For this review, take the finished solid that the model builds, in its own axes (mm). Face numbers are marked on the shaded views. A direction names the side the tool comes from. Coordinates: 2 decimals unless noted, no trailing zeros. Loops run counter-clockwise (first coordinate to the right, second up) from the corner with the lowest first, then second, coordinate; pieces in that order, holes last. Notation, with made-up numbers: M 43,26 L 98,26 A11 ccw 98,36 Z; hole C 28.5,61 d4. An arc over 180 degrees is marked long. Use one line per item in the form item = value.
```python
from build123d import *

# Parameters (mm, degrees)
F1_DEPTH = 12.7
F2_DEPTH = 25
F3_COUNT = 28
F5_R     = 0.381


with BuildPart() as f1:
    # F0 (on Top) → F1 (new body)
    with BuildSketch(Plane.XY):
        with BuildLine():
            ThreePointArc((0, 31.75), (-22.4506403027, -22.4506403027), (31.75, 0))
            ThreePointArc((31.75, 0), (24.9039389343, 19.6940682835), (7.3181054768, 30.895110167))
            Line((7.3181054768, 30.895110167), (0, 26.67))
            Line((0, 26.67), (0, 31.75))
        make_face()
        Polygon((0, 7.9189362922), (6.858, 3.9594681461), (6.858, -3.9594681461), (0, -7.9189362922), (-6.858, -3.9594681461), (-6.858, 3.9594681461), align=None, mode=Mode.SUBTRACT)
        with BuildLine():
            Line((0, 26.67), (7.3181054768, 30.895110167))
            ThreePointArc((7.3181054768, 30.895110167), (3.6839348663, 31.5355533311), (0, 31.75))
            Line((0, 31.75), (0, 26.67))
        make_face()
    extrude(amount=F1_DEPTH)


with BuildPart() as f2:
    # F0 (on Top) → F2 (new body)
    with BuildSketch(Plane.XY):
        with BuildLine():
            Line((0, 26.67), (7.3181054768, 30.895110167))
            ThreePointArc((7.3181054768, 30.895110167), (3.6839348663, 31.5355533311), (0, 31.75))
            Line((0, 31.75), (0, 26.67))
        make_face()
    extrude(amount=F2_DEPTH)


with BuildPart() as f3_1:
    # F3: instance of F2
    add(f2.part.rotate(Axis((0, 0, 0), (0, 0, -1)), 1 * 360 / F3_COUNT))


with BuildPart() as f3_2:
    # F3: instance of F2
    add(f2.part.rotate(Axis((0, 0, 0), (0, 0, -1)), 2 * 360 / F3_COUNT))


with BuildPart() as f3_3:
    # F3: instance of F2
    add(f2.part.rotate(Axis((0, 0, 0), (0, 0, -1)), 3 * 360 / F3_COUNT))


with BuildPart() as f3_4:
    # F3: instance of F2
    add(f2.part.rotate(Axis((0, 0, 0), (0, 0, -1)), 4 * 360 / F3_COUNT))


with BuildPart() as f3_5:
    # F3: instance of F2
    add(f2.part.rotate(Axis((0, 0, 0), (0, 0, -1)), 5 * 360 / F3_COUNT))


with BuildPart() as f3_6:
    # F3: instance of F2
    add(f2.part.rotate(Axis((0, 0, 0), (0, 0, -1)), 6 * 360 / F3_COUNT))


with BuildPart() as f3_7:
    # F3: instance of F2
    add(f2.part.rotate(Axis((0, 0, 0), (0, 0, -1)), 7 * 360 / F3_COUNT))


with BuildPart() as f3_8:
    # F3: instance of F2
    add(f2.part.rotate(Axis((0, 0, 0), (0, 0, -1)), 8 * 360 / F3_COUNT))


with BuildPart() as f3_9:
    # F3: instance of F2
    add(f2.part.rotate(Axis((0, 0, 0), (0, 0, -1)), 9 * 360 / F3_COUNT))


with BuildPart() as f3_10:
    # F3: instance of F2
    add(f2.part.rotate(Axis((0, 0, 0), (0, 0, -1)), 10 * 360 / F3_COUNT))


with BuildPart() as f3_11:
    # F3: instance of F2
    add(f2.part.rotate(Axis((0, 0, 0), (0, 0, -1)), 11 * 360 / F3_COUNT))


with BuildPart() as f3_12:
    # F3: instance of F2
    add(f2.part.rotate(Axis((0, 0, 0), (0, 0, -1)), 12 * 360 / F3_COUNT))


with BuildPart() as f3_13:
    # F3: instance of F2
    add(f2.part.rotate(Axis((0, 0, 0), (0, 0, -1)), 13 * 360 / F3_COUNT))


with BuildPart() as f3_14:
    # F3: instance of F2
    add(f2.part.rotate(Axis((0, 0, 0), (0, 0, -1)), 14 * 360 / F3_COUNT))


with BuildPart() as f3_15:
    # F3: instance of F2
    add(f2.part.rotate(Axis((0, 0, 0), (0, 0, -1)), 15 * 360 / F3_COUNT))


with BuildPart() as f3_16:
    # F3: instance of F2
    add(f2.part.rotate(Axis((0, 0, 0), (0, 0, -1)), 16 * 360 / F3_COUNT))


with BuildPart() as f3_17:
    # F3: instance of F2
    add(f2.part.rotate(Axis((0, 0, 0), (0, 0, -1)), 17 * 360 / F3_COUNT))


with BuildPart() as f3_18:
    # F3: instance of F2
    add(f2.part.rotate(Axis((0, 0, 0), (0, 0, -1)), 18 * 360 / F3_COUNT))


with BuildPart() as f3_19:
    # F3: instance of F2
    add(f2.part.rotate(Axis((0, 0, 0), (0, 0, -1)), 19 * 360 / F3_COUNT))


with BuildPart() as f3_20:
    # F3: instance of F2
    add(f2.part.rotate(Axis((0, 0, 0), (0, 0, -1)), 20 * 360 / F3_COUNT))


with BuildPart() as f3_21:
    # F3: instance of F2
    add(f2.part.rotate(Axis((0, 0, 0), (0, 0, -1)), 21 * 360 / F3_COUNT))


with BuildPart() as f3_22:
    # F3: instance of F2
    add(f2.part.rotate(Axis((0, 0, 0), (0, 0, -1)), 22 * 360 / F3_COUNT))


with BuildPart() as f3_23:
    # F3: instance of F2
    add(f2.part.rotate(Axis((0, 0, 0), (0, 0, -1)), 23 * 360 / F3_COUNT))


with BuildPart() as f3_24:
    # F3: instance of F2
    add(f2.part.rotate(Axis((0, 0, 0), (0, 0, -1)), 24 * 360 / F3_COUNT))


with BuildPart() as f3_25:
    # F3: instance of F2
    add(f2.part.rotate(Axis((0, 0, 0), (0, 0, -1)), 25 * 360 / F3_COUNT))


with BuildPart() as f3_26:
    # F3: instance of F2
    add(f2.part.rotate(Axis((0, 0, 0), (0, 0, -1)), 26 * 360 / F3_COUNT))


with BuildPart() as f3_27:
    # F3: instance of F2
    add(f2.part.rotate(Axis((0, 0, 0), (0, 0, -1)), 27 * 360 / F3_COUNT))


with BuildPart() as f1_1:
    add(f1.part)

    # F4: cut F2, F3_1, F3_2, F3_3, F3_4, F3_5, F3_6, F3_7, F3_8, F3_9, F3_10, F3_11, F3_12, F3_13, F3_14, F3_15, F3_16, F3_17, F3_18, F3_19, F3_20, F3_21, F3_23, F3_22, F3_24, F3_25, F3_26, F3_27
    add(f2.part, mode=Mode.SUBTRACT)
    add(f3_1.part, mode=Mode.SUBTRACT)
    add(f3_2.part, mode=Mode.SUBTRACT)
    add(f3_3.part, mode=Mode.SUBTRACT)
    add(f3_4.part, mode=Mode.SUBTRACT)
    add(f3_5.part, mode=Mode.SUBTRACT)
    add(f3_6.part, mode=Mode.SUBTRACT)
    add(f3_7.part, mode=Mode.SUBTRACT)
    add(f3_8.part, mode=Mode.SUBTRACT)
    add(f3_9.part, mode=Mode.SUBTRACT)
    add(f3_10.part, mode=Mode.SUBTRACT)
    add(f3_11.part, mode=Mode.SUBTRACT)
    add(f3_12.part, mode=Mode.SUBTRACT)
    add(f3_13.part, mode=Mode.SUBTRACT)
    add(f3_14.part, mode=Mode.SUBTRACT)
    add(f3_15.part, mode=Mode.SUBTRACT)
    add(f3_16.part, mode=Mode.SUBTRACT)
    add(f3_17.part, mode=Mode.SUBTRACT)
    add(f3_18.part, mode=Mode.SUBTRACT)
    add(f3_19.part, mode=Mode.SUBTRACT)
    add(f3_20.part, mode=Mode.SUBTRACT)
    add(f3_21.part, mode=Mode.SUBTRACT)
    add(f3_23.part, mode=Mode.SUBTRACT)
    add(f3_22.part, mode=Mode.SUBTRACT)
    add(f3_24.part, mode=Mode.SUBTRACT)
    add(f3_25.part, mode=Mode.SUBTRACT)
    add(f3_26.part, mode=Mode.SUBTRACT)
    add(f3_27.part, mode=Mode.SUBTRACT)

    # F5
    f5_edges = [f1_1.edges().sort_by_distance(p)[0] for p in [
        (-31.507862, 0, 6.35),
        (-30.717895, 7.011159, 6.35),
        (-28.387603, 13.670749, 6.35),
        (-24.633839, 19.644831, 6.35),
        (-19.644831, 24.633839, 6.35),
        (-13.670749, 28.387603, 6.35),
        (-7.011159, 30.717895, 6.35),
        (0, 31.507862, 6.35),
        (7.011159, 30.717895, 6.35),
        (13.670749, 28.387603, 6.35),
        (19.644831, 24.633839, 6.35),
        (24.633839, 19.644831, 6.35),
        (28.387603, 13.670749, 6.35),
        (30.717895, 7.011159, 6.35),
        (31.507862, 0, 6.35),
        (30.717895, -7.011159, 6.35),
        (28.387603, -13.670749, 6.35),
        (24.633839, -19.644831, 6.35),
        (19.644831, -24.633839, 6.35),
        (13.670749, -28.387603, 6.35),
        (7.011159, -30.717895, 6.35),
        (0, -31.507862, 6.35),
        (-7.011159, -30.717895, 6.35),
        (-13.670749, -28.387603, 6.35),
        (-19.644831, -24.633839, 6.35),
        (-24.633839, -19.644831, 6.35),
        (-28.387603, -13.670749, 6.35),
        (-30.717895, -7.011159, 6.35),
        (26.001327, 5.934633, 6.35),
        (26.67, 0, 6.35),
        (26.001327, -5.934633, 6.35),
        (24.02884, -11.571679, 6.35),
        (20.851446, -16.628473, 6.35),
        (16.628473, -20.851446, 6.35),
        (11.571679, -24.02884, 6.35),
        (5.934633, -26.001327, 6.35),
        (0, -26.67, 6.35),
        (-5.934633, -26.001327, 6.35),
        (-11.571679, -24.02884, 6.35),
        (-16.628473, -20.851446, 6.35),
        (-20.851446, -16.628473, 6.35),
        (-24.02884, -11.571679, 6.35),
        (-26.001327, -5.934633, 6.35),
        (-26.67, 0, 6.35),
        (-26.001327, 5.934633, 6.35),
        (-24.02884, 11.571679, 6.35),
        (-20.851446, 16.628473, 6.35),
        (-16.628473, 20.851446, 6.35),
        (-11.571679, 24.02884, 6.35),
        (-5.934633, 26.001327, 6.35),
        (0, 26.67, 6.35),
        (5.934633, 26.001327, 6.35),
        (11.571679, 24.02884, 6.35),
        (16.628473, 20.851446, 6.35),
        (20.851446, 16.628473, 6.35),
        (24.02884, 11.571679, 6.35),
    ]]
    fillet(f5_edges, radius=F5_R)


solid = f1_1.part
```
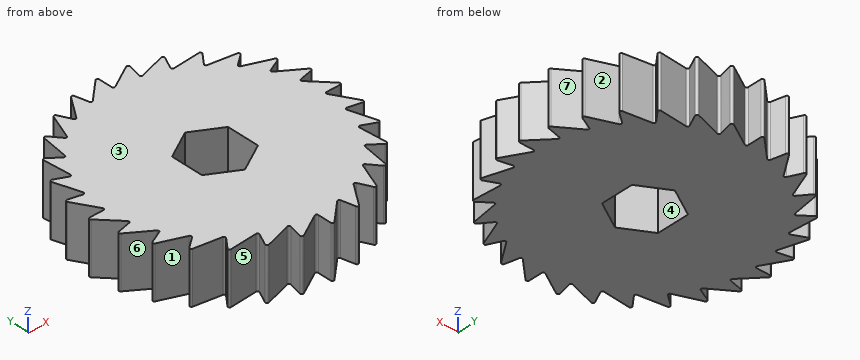
1. Consider section B-B on x = 3. Write out the cut boundary in (y, z), plus the area to 3 significant figures.
Computed values:
outline = M -28.72,0 L -6.19,0 L -6.19,12.7 L -28.72,12.7 Z; M 6.19,0 L 28.4,0 L 28.4,12.7 L 6.19,12.7 Z
area = 568 mm2
2. Consider section C-C on x = -9. Write out the cut boundary in (y, z).
Computed values:
outline = M -26.95,0 L 27.8,0 L 27.8,12.7 L -26.95,12.7 Z
3. For pin 1 Ø3.5 at (y, z) = (28.5, 8.5) entering from +X; pin 2 Ø2.5 at (y, z) = (-1.5, 4.5) entering from +X; pin 3 Ø2.5 at (y, z) = (1.5, 3.5) entering from -X, all flat-tipped, find the tip position at first contact; note any pin that passes through.
Computed values:
pin_1 = 13.33
pin_2 = 28.26
pin_3 = -28.26
4. Draft analysis for pull direction X (two halves, no side actions). For the marked faces 1, 2, 3 and 4, state which applies: +X half, -X half, draft (parallel to the pull), parting line (faces both ways), or undercut.
Computed values:
face_1 = -X half
face_2 = +X half
face_3 = draft
face_4 = undercut
5. Wall thickness on line 1 along Y through (x, z) = (-26, 9); line 2 along Y through (x, z) = (1.5, 7.25); line 3 along X through (y, z) = (-3.5, 11.75): over which ranges is each line inside the solid? List them lowest first. Write a range as from..to.
Computed values:
line_1 = -14.61..-12.52, -10.23..12.52
line_2 = -30.12..-7.05, 7.05..27.54
line_3 = -28.26..-6.86, 6.86..28.69
6. Tool access review of the marked faces 5, 6 and 7: name each direction out of +Z, -Z, +X, -X, +Y, -Y from which nothing blocks a thin tool from reaching the whole face with its end or side.
Computed values:
face_5 = +Z, -Z
face_6 = +Z, -Z, -X
face_7 = +Z, -Z, +X
7. Consider section A-A on y = 2. Write out the cut boundary in (x, z).
Computed values:
outline = M -27.82,0 L -6.86,0 L -6.86,12.7 L -27.82,12.7 Z; M 6.86,0 L 29.65,0 L 29.65,12.7 L 6.86,12.7 Z
